The drawing under review shows one solid part. Ordinate dimensions are in mm from its lowest x, y, z. A direction names the side the tool comes from. Round coordinates to 2 decimals unless told otherwise and drop trailing zeros. Order: outer loops, then holes, each group sorted by start corner. A loop starts at its lowest first (then second) coordinate and runs counter-clockwise, first axis right, second up. Notation, with made-up numbers: (-39.5, 57.5) -> (4.5, 57.5) arc R19 cw to (4.5, 78.5) -> close; hole circle Ø7 at (88, 83.5). An arc over 180 degrees is marked (long way). Use a Markdown table: item, result. Add a question column.
1) Machinability: for the marked faces 1 and 2, which of the approach directions +Z, -Z, +X, -X, +Y, -Y give a long, thin tool a straight path to every point of the face, cutting with its end or side? Answer none if there is none.
2) Consider section B-B (x = 59.5). State the section outline as (y, z) points.
3) Consider section A-A (z = 99.5). State the section outline as (x, y) points, plus the area to 3 significant figures.
4) Draft analysis for pull direction Y (two halves, no side actions). For the marked faces 3, 4 and 5, state which applies: pulls with the +Y half, pulls with the -Y half, needs draft (parallel to the pull), parting line crosses it, or undercut.
5) Consider section D-D (x = 125). State the section outline as (y, z) points, plus the area to 3 significant figures.
6) Wall thickness on line 1 along X through (y, z) = (16, 98); line 2 along X through (y, z) = (46.5, 107.5) (1 decimal); line 3 along X through (y, z) = (67.5, 147) (1 decimal): over which ranges is each line inside the solid? List them lowest first. Write a range as [from, to].
7) Clearance check with flat-ended pins moving along their axes: P1, Ø8, axis at x = 71, z = 46, coming from the -Y side; P2, Ø3, axis at y = 67.5, z = 48.5, coming from the +X side; P3, Ø2, axis at x = 147.5, z = 41.5, coming from the -Y side. State where each tip first meets the part, or that it passes through.
8) Consider section C-C (y = 52). State the section outline as (x, z) points.
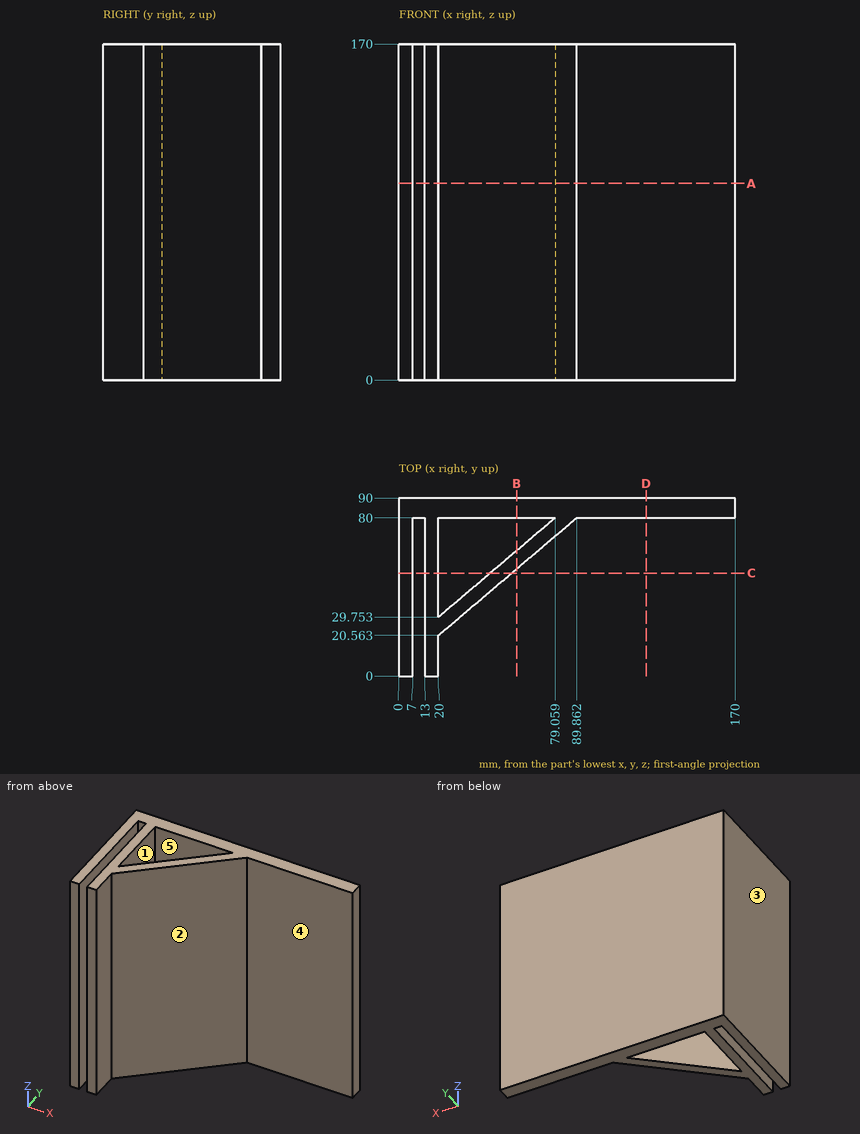
Results list:
| question | item | result |
|---|---|---|
| 1 | face 1 | +Z, -Z |
| 1 | face 2 | +Z, -Z, +X, -Y |
| 2 | outline | (54.17, 0) -> (63.36, 0) -> (63.36, 170) -> (54.17, 170) -> close; (80, 0) -> (90, 0) -> (90, 170) -> (80, 170) -> close |
| 3 | outline | (0, 0) -> (7, 0) -> (7, 80) -> (13, 80) -> (13, 0) -> (20, 0) -> (20, 20.56) -> (89.86, 80) -> (170, 80) -> (170, 90) -> (0, 90) -> close; hole (20, 29.75) -> (79.06, 80) -> (20, 80) -> close |
| 3 | area | 3,410 mm2 |
| 4 | face 3 | needs draft |
| 4 | face 4 | pulls with the -Y half |
| 4 | face 5 | undercut |
| 5 | outline | (80, 0) -> (90, 0) -> (90, 170) -> (80, 170) -> close |
| 5 | area | 1,700 mm2 |
| 6 | line 1 | [0, 7], [13, 20] |
| 6 | line 2 | [0, 7], [13, 20], [39.7, 50.5] |
| 6 | line 3 | [0, 7], [13, 20], [64.4, 75.2] |
| 7 | P1 | y = 60.55 |
| 7 | P2 | x = 76.93 |
| 7 | P3 | y = 80 |
| 8 | outline | (0, 0) -> (7, 0) -> (7, 170) -> (0, 170) -> close; (13, 0) -> (20, 0) -> (20, 170) -> (13, 170) -> close; (46.15, 0) -> (56.95, 0) -> (56.95, 170) -> (46.15, 170) -> close |
